Source: CAD feature listing. Evaluate the final solid. Frame: model axes, mm. Coordinates: 2 decimals unless noted, no trailing zeros. Write each loop counter-clockwise with the first axis right and the second up, starting at its lowest first coordinate (ties: lowest second). Pieces come first, ordered by that corner, then holes. Notation, with made-up numbers: (57, 79.5) - (105, 79.5) arc R26 cw to (105, 97.5) - close; hole circle Ø1 at (-19.5, -32). An arc over 180 degrees is marked (long way). One line per question, with ' | ' between items.
from build123d import *

# Parameters (mm, degrees)
F0_W        = 88.9
F0_H        = 254
F1_DEPTH    = 2.54
F2_T1_DEPTH = 127
F2_T3_DEPTH = 292.1
F5_D        = 2.54
F5_DEPTH    = 5.08
F5_TIP      = 0.7630929862


# Not quite as in the source:
# - a fillet or chamfer that OpenCascade refuses, or shapes differently, is made with other operations: its cross-section is extruded or revolved along the edge and cut away or added


with BuildPart() as f1:
    # F0 (on Top) → F1 (new body)
    with BuildSketch(Plane.XY):
        Rectangle(F0_W, F0_H)
    extrude(amount=F1_DEPTH)

    # F2: fillet of radius 12.7 on 4 edges, made by hand

    # F2_s2 → F2_t1 (cut)
    with BuildSketch(Plane.YZ.offset(-63.5)):
        with BuildLine():
            ThreePointArc((127, 0), (123.3960926284, 1.8882778852), (119.38, 2.54))
            Line((119.38, 2.54), (127, 2.54))
            Line((127, 2.54), (127, 0))
        make_face()
        with BuildLine():
            ThreePointArc((-127, 0), (-123.3960926284, 1.8882778852), (-119.38, 2.54))
            Line((-119.38, 2.54), (-127, 2.54))
            Line((-127, 2.54), (-127, 0))
        make_face()
    extrude(amount=F2_T1_DEPTH, mode=Mode.SUBTRACT)

    # F2_s4 → F2_t3 (cut)
    with BuildSketch(Plane.XZ.offset(-146.05)):
        with BuildLine():
            ThreePointArc((-44.45, 0), (-40.8460926284, 1.8882778852), (-36.83, 2.54))
            Line((-36.83, 2.54), (-44.45, 2.54))
            Line((-44.45, 2.54), (-44.45, 0))
        make_face()
        with BuildLine():
            ThreePointArc((44.45, 0), (40.8460926284, 1.8882778852), (36.83, 2.54))
            Line((36.83, 2.54), (44.45, 2.54))
            Line((44.45, 2.54), (44.45, 0))
        make_face()
    extrude(amount=F2_T3_DEPTH, mode=Mode.SUBTRACT)

    # F5
    with Locations(Plane.XY.offset(2.54)):
        with Locations((-28.8370940834, 104.9257144332), (28.5376422107, 104.9257144332), (28.5376422107, 0), (-28.8370940834, 0), (-28.8370940834, -104.8506721854), (28.5376422107, -104.4920757413)):
            Hole(F5_D / 2, depth=F5_DEPTH)
            with Locations((0, 0, -(F5_DEPTH + F5_TIP / 2))):  # 118° drill point
                Cone(0, F5_D / 2, F5_TIP, mode=Mode.SUBTRACT)


solid = f1.part
Item 1: Cut plane A-A on z = 1.65. Return loops of the section in (x, y).
Check sheet entries:
outline: (-41.5, -124.05) - (41.5, -124.05) - (41.5, 124.05) - (-41.5, 124.05) - close; hole circle Ø2.54 at (-28.84, -104.85); hole circle Ø2.54 at (-28.84, 0); hole circle Ø2.54 at (-28.84, 104.93); hole circle Ø2.54 at (28.54, -104.49); hole circle Ø2.54 at (28.54, 0); hole circle Ø2.54 at (28.54, 104.93)
Item 2: Cut plane C-C on y = -89. Return loops of the section in (x, z).
Check sheet entries:
outline: (-44.45, 0) - (44.45, 0) arc R12.7 ccw to (36.83, 2.54) - (-36.83, 2.54) arc R12.7 ccw to start
Item 3: Cut plane B-B on x = -10.5. Return loops of the section in (y, z), and give its area (3 significant figures).
Check sheet entries:
outline: (-127, 0) - (127, 0) arc R12.7 ccw to (119.38, 2.54) - (-119.38, 2.54) arc R12.7 ccw to start | area: 633 mm²
Item 4: Ray query, line 1 along X through (y, z) = (45, 0.25); line 2 along Y through (x, z) = (-23, 1.15); line 3 along X through (y, z) = (-94.5, 1.1). Return the intervals inside material, ascending. Write a range as [from, to].
Check sheet entries:
line 1: [-44.1, 44.1] | line 2: [-125.16, 125.16] | line 3: [-42.7, 42.7]
Item 5: Pin query (flat end, axial travel): pin 1 Ø1.5 at (x, y) = (28.54, -104.49) entering from +Z. Return the tip coordinate at first contact, or that it passes through.
Check sheet entries:
pin 1: through
